Part model, mm, in its own coordinate system. A direction names the side the tool comes from. Coordinates: 2 decimals unless noted, no trailing zeros. Write each loop counter-clockwise with the first axis right and the second up, starting at its lowest first coordinate (ties: lowest second). Pieces come first, ordered by that corner, then holes. Notation, with made-up numbers: (79, 19.5) - (136, 19.5) arc R27 ccw to (136, 55.5) - close; hole circle Ø8 at (45.5, 61.5). An arc over 180 degrees is marked (long way). Use a Markdown table: item, result.
```python
from build123d import *

# Parameters (mm, degrees)
BOSS_EXTRUDE1_DEPTH           = 7.5
FILLET1_R                     = 2
FILLET2_R                     = 5
CHAMFER1_SIZE                 = 1
M2_5_TAPPED_HOLE1_D           = 2.4
M2_5_TAPPED_HOLE1_CSINK_D     = 3
M2_5_TAPPED_HOLE1_CSINK_ANGLE = 90


with BuildPart() as part:
    # Sketch1 → Boss-Extrude1 (new body, symmetric)
    with BuildSketch(Plane.XY):
        with BuildLine():
            Line((10.96838323, -65.321653098), (44.869098301, -14.095171079))
            ThreePointArc((44.869098301, -14.095171079), (48.66504531, -14.940478439), (52.550723574, -14.781536092))
            Line((52.550723574, -14.781536092), (56.963282689, -22.992992284))
            ThreePointArc((56.963282689, -22.992992284), (58.445062856, -24.203567674), (60.348845726, -24.011796937))
            Line((60.348845726, -24.011796937), (64.312776647, -21.88171439))
            ThreePointArc((64.312776647, -21.88171439), (65.523352037, -20.399934224), (65.331581299, -18.496151353))
            Line((65.331581299, -18.496151353), (60.919022184, -10.284695161))
            ThreePointArc((60.919022184, -10.284695161), (63.213103069, 7.100275156), (47.449276426, 14.781536092))
            Line((47.449276426, 14.781536092), (43.036717311, 22.992992284))
            ThreePointArc((43.036717311, 22.992992284), (41.554937144, 24.203567674), (39.651154274, 24.011796937))
            Line((39.651154274, 24.011796937), (35.687223353, 21.88171439))
            ThreePointArc((35.687223353, 21.88171439), (34.476647963, 20.399934224), (34.668418701, 18.496151353))
            Line((34.668418701, 18.496151353), (39.080977816, 10.284695161))
            ThreePointArc((39.080977816, 10.284695161), (36.804017619, 7.132043817), (35.414047854, 3.5))
            Line((35.414047854, 3.5), (-35.414047854, 3.5))
            ThreePointArc((-35.414047854, 3.5), (-36.804017619, 7.132043817), (-39.080977816, 10.284695161))
            Line((-39.080977816, 10.284695161), (-34.668418701, 18.496151353))
            ThreePointArc((-34.668418701, 18.496151353), (-34.476647963, 20.399934224), (-35.687223353, 21.88171439))
            Line((-35.687223353, 21.88171439), (-39.651154274, 24.011796937))
            ThreePointArc((-39.651154274, 24.011796937), (-41.554937144, 24.203567674), (-43.036717311, 22.992992284))
            Line((-43.036717311, 22.992992284), (-47.449276426, 14.781536092))
            ThreePointArc((-47.449276426, 14.781536092), (-63.213103069, 7.100275156), (-60.919022184, -10.284695161))
            Line((-60.919022184, -10.284695161), (-65.331581299, -18.496151353))
            ThreePointArc((-65.331581299, -18.496151353), (-65.523352037, -20.399934224), (-64.312776647, -21.88171439))
            Line((-64.312776647, -21.88171439), (-60.348845726, -24.011796937))
            ThreePointArc((-60.348845726, -24.011796937), (-58.445062856, -24.203567674), (-56.963282689, -22.992992284))
            Line((-56.963282689, -22.992992284), (-52.550723574, -14.781536092))
            ThreePointArc((-52.550723574, -14.781536092), (-48.66504531, -14.940478439), (-44.869098301, -14.095171079))
            Line((-44.869098301, -14.095171079), (-10.96838323, -65.321653098))
            ThreePointArc((-10.96838323, -65.321653098), (0, -90.553689519), (10.96838323, -65.321653098))
        make_face()
        with BuildLine():
            Line((39.03161677, -10.232036421), (23.460950184, -33.760462599))
            Line((23.460950184, -33.760462599), (2.5, -19.888902972))
            Line((2.5, -19.888902972), (2.5, -3.5))
            Line((2.5, -3.5), (35.414047854, -3.5))
            ThreePointArc((35.414047854, -3.5), (36.786896931, -7.100275156), (39.03161677, -10.232036421))
        make_face(mode=Mode.SUBTRACT)
        with BuildLine():
            Line((-35.414047854, -3.5), (-2.5, -3.5))
            Line((-2.5, -3.5), (-2.5, -19.888902972))
            Line((-2.5, -19.888902972), (-23.460950184, -33.760462599))
            Line((-23.460950184, -33.760462599), (-39.03161677, -10.232036421))
            ThreePointArc((-39.03161677, -10.232036421), (-36.786896931, -7.100275156), (-35.414047854, -3.5))
        make_face(mode=Mode.SUBTRACT)
        with BuildLine():
            Line((-20.701568286, -37.930092263), (0, -24.230186661))
            Line((0, -24.230186661), (20.701568286, -37.930092263))
            Line((20.701568286, -37.930092263), (5.130901699, -61.45851844))
            ThreePointArc((5.130901699, -61.45851844), (0, -60.553689519), (-5.130901699, -61.45851844))
            Line((-5.130901699, -61.45851844), (-20.701568286, -37.930092263))
        make_face(mode=Mode.SUBTRACT)
    extrude(amount=BOSS_EXTRUDE1_DEPTH, both=True)

    # Fillet1
    fillet1_edges = [part.edges().sort_by_distance(p)[0] for p in [
        (-35.414047854, -3.5, 0),
        (-39.03161677, -10.232036421, 0),
        (-23.460950184, -33.760462599, 0),
        (-2.5, -19.888902972, 0),
        (-2.5, -3.5, 0),
        (-52.550723574, -14.781536092, 0),
        (-60.919022184, -10.284695161, 0),
        (-47.449276426, 14.781536092, 0),
        (-39.080977816, 10.284695161, 0),
        (39.080977816, 10.284695161, 0),
        (47.449276426, 14.781536092, 0),
        (60.919022184, -10.284695161, 0),
        (52.550723574, -14.781536092, 0),
        (39.03161677, -10.232036421, 0),
        (35.414047854, -3.5, 0),
        (2.5, -3.5, 0),
        (2.5, -19.888902972, 0),
        (23.460950184, -33.760462599, 0),
        (-5.130901699, -61.45851844, 0),
        (5.130901699, -61.45851844, 0),
        (20.701568286, -37.930092263, 0),
        (0, -24.230186661, 0),
        (-20.701568286, -37.930092263, 0),
    ]]
    fillet(fillet1_edges, radius=FILLET1_R)

    # Fillet2
    fillet2_edges = [part.edges().sort_by_distance(p)[0] for p in [
        (-10.96838323, -65.321653098, 0),
        (-44.869098301, -14.095171079, 0),
        (-35.414047854, 3.5, 0),
        (35.414047854, 3.5, 0),
        (44.869098301, -14.095171079, 0),
        (10.96838323, -65.321653098, 0),
    ]]
    fillet(fillet2_edges, radius=FILLET2_R)

    # Sketch6 → Cut-Revolve1 (revolve, cut)
    with BuildSketch(Plane(origin=(-50, 0, 0), x_dir=(0, 0, -1), z_dir=(1, 0, 0))):
        Polygon((-7.5, 0), (-7.5, 7.5), (-2.5, 7.5), (-2.5, 9.5), (7.5, 9.5), (7.5, 0), align=None)
    revolve(axis=Axis((-50, 0, 7.5), (0, 0, -1)), mode=Mode.SUBTRACT)

    # Sketch7 → Cut-Revolve2 (revolve, cut)
    with BuildSketch(Plane(origin=(50, 0, 0), x_dir=(0, 0, -1), z_dir=(1, 0, 0))):
        Polygon((7.5, 0), (-7.5, 0), (-7.5, 7.5), (-2.5, 7.5), (-2.5, 9.5), (7.5, 9.5), align=None)
    revolve(axis=Axis((50, 0, 7.5), (0, 0, -1)), mode=Mode.SUBTRACT)

    # Sketch8 → Cut-Revolve3 (revolve, cut)
    with BuildSketch(Plane(origin=(0, 0, 0), x_dir=(0, 0, -1), z_dir=(1, 0, 0))):
        Polygon((7.5, -75.553689519), (-15.002177418, -75.553689519), (-7.5, -83.053689519), (-2.5, -83.053689519), (-2.5, -85.053689519), (7.5, -85.053689519), align=None)
    revolve(axis=Axis((0, -75.553689519, 7.5), (0, 0, -1)), mode=Mode.SUBTRACT)

    # Chamfer1
    chamfer1_edges = [part.edges().sort_by_distance(p)[0] for p in [
        (-50, -9.5, -7.5),
        (50, -9.5, -7.5),
        (0, -66.053689519, -7.5),
    ]]
    chamfer(chamfer1_edges, length=CHAMFER1_SIZE)

    # M2.5 Tapped Hole1 (through all)
    with Locations(Plane(origin=(0, 0, -7.5), x_dir=(-1, 0, 0), z_dir=(0, 0, -1))):
        with Locations((-39.112911428, 20.260091373), (-60.887088572, -20.260091373), (39.112911428, 20.260091373), (60.887088572, -20.260091373)):
            CounterSinkHole(M2_5_TAPPED_HOLE1_D / 2, M2_5_TAPPED_HOLE1_CSINK_D / 2, counter_sink_angle=M2_5_TAPPED_HOLE1_CSINK_ANGLE)


solid = part.part
```
Item 1: Band-saw the part on B-B, the plane y = -29. Give the cut face in (x, z), then the cut area to 3 significant figures.
From the geometry:
| item | result |
|---|---|
| outline | (-35.01, -7.5) - (-26.61, -7.5) - (-26.61, 7.5) - (-35.01, 7.5) - close; (-16.27, -7.5) - (-7.21, -7.5) - (-7.21, 7.5) - (-16.27, 7.5) - close; (7.21, -7.5) - (16.27, -7.5) - (16.27, 7.5) - (7.21, 7.5) - close; (26.61, -7.5) - (35.01, -7.5) - (35.01, 7.5) - (26.61, 7.5) - close |
| area | 524 mm^2 |
Item 2: Band-saw the part on D-D, the plane z = -4.5. Count the separate pieces of the cut face and the enclosed holes in it, then the cut area to 3 significant figures.
From the geometry:
| item | result |
|---|---|
| separate pieces | 1 |
| enclosed holes | 10 |
| area | 3,380 mm^2 |
Item 3: Drop flat-ended pins along their axis: P1, Ø9.5, axis at x = -52.5, y = 2.5, coming from the -Z side; P2, Ø10, axis at x = 24.5, y = 10, coming from the +Z side; P3, Ø4, axis at x = -60.89, y = -20.26, coming from the -Z side; P4, Ø1.5, axis at y = -51.5, z = -4, coming from the -X side. Give the stop position or say it passes through.
From the geometry:
| item | result |
|---|---|
| P1 | z = 2.5 |
| P2 | through |
| P3 | z = -7.5 |
| P4 | x = -20.61 |
Item 4: Drill centre lines: probe 1 along Y at (x, z) = (0, -3.25); probe 2 along X at (y, z) = (0, 6.3); probe 3 along X at (y, z) = (0, -4.5). Where is each one in solid material? Low to high.
From the geometry:
| item | result |
|---|---|
| probe 1 | -90.55 to -85.05, -66.05 to -60.55, -24.63 to 3.5 |
| probe 2 | -65 to -57.5, -42.5 to 42.5, 57.5 to 65 |
| probe 3 | -65 to -59.5, -40.5 to 40.5, 59.5 to 65 |
Item 5: Two-plate mould, pull along Y, no slides. Class faces 1 (the face through (58.419, -24.196, 0.105)), 2 (the face through (-65.531, -20.374, 0.105)), 3 (the face through (36.523, 15.045, 0.105)): pulls with the +Y half, pulls with the -Y half, needs draft (parallel to the pull), parting line crosses it, or undercut.
From the geometry:
| item | result |
|---|---|
| face 1 | pulls with the -Y half |
| face 2 | parting line crosses it |
| face 3 | undercut |
Item 6: Which spindle directions (+Z, -Z, +X, -X, +Y, -Y) get a long thin tool onto all of the face, cutting with end or side? Do faces 4 (the face through (-37.23, 7.87, 0.11)), 5 (the face through (-37.64, 22.93, 0.11)), 6 (the face through (58, -1, 2.5)), 7 (the face through (-63.4, -14.9, 0.1)). Say none if no direction does.
From the geometry:
| item | result |
|---|---|
| face 4 | +Z, -Z |
| face 5 | +Z, -Z, +Y |
| face 6 | -Z |
| face 7 | +Z, -Z, -X |
Item 7: Band-saw the part on C-C, the plane y = -44. Give the cut face in (x, z), then the cut area to 3 significant figures.
From the geometry:
| item | result |
|---|---|
| outline | (-25.08, -7.5) - (-16.68, -7.5) - (-16.68, 7.5) - (-25.08, 7.5) - close; (16.68, -7.5) - (25.08, -7.5) - (25.08, 7.5) - (16.68, 7.5) - close |
| area | 252 mm^2 |
Item 8: Band-saw the part on A-A, the plane y = 0. Give the cut face in (x, z), then the cut area to 3 significant figures.
From the geometry:
| item | result |
|---|---|
| outline | (-65, -7.5) - (-60.5, -7.5) - (-59.5, -6.5) - (-59.5, 2.5) - (-57.5, 2.5) - (-57.5, 7.5) - (-65, 7.5) - close; (-42.5, 2.5) - (-40.5, 2.5) - (-40.5, -6.5) - (-39.5, -7.5) - (39.5, -7.5) - (40.5, -6.5) - (40.5, 2.5) - (42.5, 2.5) - (42.5, 7.5) - (-42.5, 7.5) - close; (57.5, 2.5) - (59.5, 2.5) - (59.5, -6.5) - (60.5, -7.5) - (65, -7.5) - (65, 7.5) - (57.5, 7.5) - close |
| area | 1,420 mm^2 |
